Check sheet for the modelled part. Datum: model origin and axes. Units: mm. Face numbers are marked on the shaded views. A direction names the side the tool comes from. Coordinates: 2 decimals unless noted, no trailing zeros. Write each loop counter-clockwise with the first axis right and the second up, starting at its lowest first coordinate (ties: lowest second). Pieces come first, ordered by that corner, then holes. Notation, with made-up numbers: M 46.5,38.25 L 102.5,38.25 A35 cw 102.5,70.25 Z; hole C 65.5,59 d3. An arc over 180 degrees is marked long. Answer as CSV lines item,"result".
from build123d import *
from build123d.topology import SkipClean

# Parameters (mm, degrees)
BOSS_EXTRUDE3_DEPTH = 5
BOSS_EXTRUDE4_DEPTH = 36
SKETCH5_R           = 6
BOSS_EXTRUDE5_DEPTH = 8
SKETCH6_R           = 15
SKETCH6_R_2         = 6
BOSS_EXTRUDE6_DEPTH = 5
FILLET1_R           = 12
SKETCH8_R           = 5.1
CUT_EXTRUDE1_DEPTH  = 78.491935064
CHAMFER1_SIZE       = 0.5


with BuildPart() as part:
    # Sketch3 → Boss-Extrude3 (new, symmetric)
    with BuildSketch(Plane.XY):
        Polygon((0, 0), (0, 40), (22, 0), align=None)
    extrude(amount=BOSS_EXTRUDE3_DEPTH, both=True)

    # Sketch4 → Boss-Extrude4 (add, symmetric)
    with BuildSketch(Plane.XY):
        Polygon((22, 0), (-8, 0), (-8, -4), (-13, -4), (-13, -10), (22, -10), align=None)
    extrude(amount=BOSS_EXTRUDE4_DEPTH, both=True)

    # Sketch5 → Boss-Extrude5 (add)
    with BuildSketch(Plane(origin=(0, 0, 0), x_dir=(0, 0, -1), z_dir=(1, 0, 0))):
        with BuildLine():
            Line((-30, 0), (30, 0))
            ThreePointArc((30, 0), (19.393398282, 4.393398282), (15, 15))
            Line((15, 15), (15, 50))
            ThreePointArc((15, 50), (0, 65), (-15, 50))
            Line((-15, 50), (-15, 15))
            ThreePointArc((-15, 15), (-19.393398282, 4.393398282), (-30, 0))
        make_face()
        with Locations((0, 50)):
            Circle(SKETCH5_R, mode=Mode.SUBTRACT)
    extrude(amount=-BOSS_EXTRUDE5_DEPTH)

    # Sketch6 → Boss-Extrude6 (add)
    with SkipClean():  # the faces are left unmerged after this step: merging them gives an invalid solid
        with BuildSketch(Plane.ZY.offset(8)):
            with Locations((0, 50)):
                Circle(SKETCH6_R)
            with Locations(Location((0, 50, 0), (0, 0, 180))):
                Circle(SKETCH6_R_2, mode=Mode.SUBTRACT)
        extrude(amount=BOSS_EXTRUDE6_DEPTH)
    add(part.part.scale(1), mode=Mode.REPLACE)  # the faces are merged on a copy

    # Fillet1
    fillet1_edges = [part.edges().sort_by_distance(p)[0] for p in [
        (22, -5, -36),
        (22, -5, 36),
    ]]
    fillet(fillet1_edges, radius=FILLET1_R)

    # Sketch8 → Cut-Extrude1 (cut, through all)
    with SkipClean():  # the faces are left unmerged after this step: merging them gives an invalid solid
        with BuildSketch(Plane(origin=(0, 0, 0), x_dir=(1, 0, 0), z_dir=(0, 1, 0))):
            with Locations(Location((10, 24, 0), (0, 0, 180))):
                Circle(SKETCH8_R)
            with Locations(Location((10, -24, 0), (0, 0, 180))):
                Circle(SKETCH8_R)
        extrude(amount=-CUT_EXTRUDE1_DEPTH, mode=Mode.SUBTRACT)

    # Chamfer1
    chamfer1_edges = [part.edges().sort_by_distance(p)[0] for p in [
        (15.1, 0, -24),
        (15.1, 0, 24),
    ]]
    chamfer(chamfer1_edges, length=CHAMFER1_SIZE)


solid = part.part
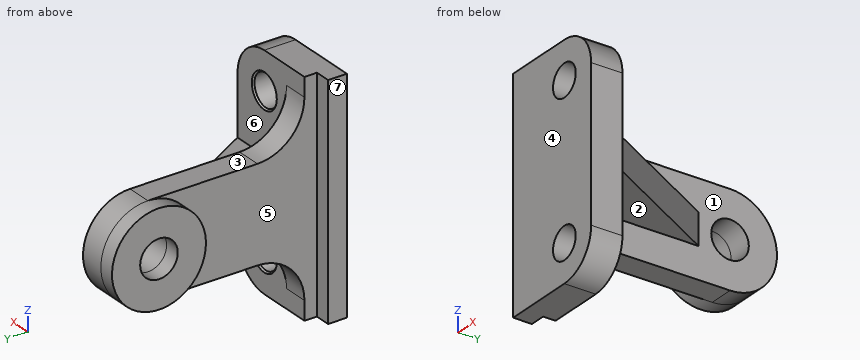
1) Depth check by flat-ended pin: P1, Ø1.5, axis at x = -10.5, z = 9, coming from the +Y side; P2, Ø9, axis at x = 5.5, z = 19, coming from the +Y side; P3, Ø4, axis at x = -3.5, y = 7.5, coming from the +Z side. Enter the tip coordinate at first touch or a pass-through.
Answer key:
P1,"stops at y = 62.53"
P2,"stops at y = 0"
P3,"stops at z = 18.39"
2) Section check D-D, the plane x = 19. Record the boundary of the cut face in (y, z).
Answer key:
outline,"M -10,-31.94 L 0,-31.94 L 0,-5 L 5.45,-5 L 5.45,5 L 0,5 L 0,31.94 L -10,31.94 Z"
3) Section check A-A, the plane z = 0. Record the boundary of the cut face in (x, y).
Answer key:
outline,"M -13,-10 L 22,-10 L 22,0 L 0,40 L 0,44 L -13,44 L -13,35 L -8,35 L -8,-4 L -13,-4 Z; M -13,56 L 0,56 L 0,65 L -13,65 Z"
4) Section check B-B, the plane x = -2.5. Record the boundary of the cut face in (y, z).
Answer key:
outline,"M -10,-36 L 0,-36 L 0,-30 A15 cw 15,-15 L 50,-15 A15 ccw 50,15 L 15,15 A15 cw 0,30 L 0,36 L -10,36 Z; hole C 50,0 d12"
5) Mould release check, pull along Y, two halves, no side actions. Record for the marked faces 4, 5, 6 and 7: pulls with the +Y half, pulls with the -Y half, needs draft (parallel to the pull), parting line crosses it, or undercut.
Answer key:
face 4,"pulls with the -Y half"
face 5,"undercut"
face 6,"pulls with the +Y half"
face 7,"needs draft"
6) Section check C-C, the plane y = 45. Record the boundary of the cut face in (x, z), plus the area to 3 significant figures.
Answer key:
outline,"M -13,-14.14 L -8,-14.14 L -8,-15 L 0,-15 L 0,-3.32 L -13,-3.32 Z; M -13,3.32 L 0,3.32 L 0,15 L -8,15 L -8,14.14 L -13,14.14 Z"
area,"295 mm2"
7) Tool access check on the marked faces 1, 2 and 3. Record the directions out of +Z, -Z, +X, -X, +Y, -Y that give a thin tool (end or side, any length) a straight path to the whole face; none if there is none.
Answer key:
face 1,"+X, +Y"
face 2,"-Z, +X, +Y"
face 3,"+Z, +X, -X, +Y"
8) Thickness scan on line 1 along Y through (x, z) = (-9.5, -3.5); line 2 along Y through (x, z) = (3.5, 14); line 3 along X through (y, z) = (51.5, 8.5). Record the ranges inside material, lowest first.
Answer key:
line 1,"y = -10 to -4, 35.41 to 45.13, 54.87 to 64.59"
line 2,"y = -10 to 0"
line 3,"x = -13 to 0"
